from build123d import *

# Parameters (mm, degrees)
SKETCH_R        = 1.75
PAD_DEPTH       = 3.05
SKETCH001_W     = 60.21645
SKETCH001_H     = 13.401505
POCKET_DEPTH    = 2.9
POCKET001_DEPTH = 3.051
POCKET002_DEPTH = 36.525
FILLET_R        = 6


with BuildPart() as part:
    # Sketch → Pad (new body)
    with BuildSketch(Plane.XY):
        Polygon((-30, 0), (30, 0), (30, 12.7), (6.524, 12.7), (6.524, 19.05), (2.968, 19.05), (2.968, 12.7), (1.778, 12.7), (1.778, 19.05), (-1.778, 19.05), (-1.778, 12.7), (-2.968, 12.7), (-2.968, 19.05), (-6.524, 19.05), (-6.524, 12.7), (-30, 12.7), align=None)
        with Locations((-24, 6.35)):
            Circle(SKETCH_R, mode=Mode.SUBTRACT)
        with Locations((24, 6.35)):
            Circle(SKETCH_R, mode=Mode.SUBTRACT)
    extrude(amount=PAD_DEPTH)

    # Sketch001 (on Face20 of Pad) → Pocket (cut)
    with BuildSketch(Plane.XY.offset(3.05)):
        with Locations((-0.108225, 5.999248)):
            Rectangle(SKETCH001_W, SKETCH001_H)
    extrude(amount=-POCKET_DEPTH, mode=Mode.SUBTRACT)

    # Sketch002 (on Face25 of Pocket) → Pocket001 (cut, through all)
    with BuildSketch(Plane.XY.offset(3.05)):
        with BuildLine():
            ThreePointArc((-2.968, 17.272), (-4.746, 19.05), (-6.524, 17.272))
            Line((-6.524, 17.272), (-7.554864, 19.132154))
            Line((-7.554864, 19.132154), (-6.342233, 20.53426))
            Line((-6.342233, 20.53426), (5.632503, 20.53426))
            Line((5.632503, 20.53426), (7.211451, 19.637419))
            Line((6.524, 17.272), (7.211451, 19.637419))
            ThreePointArc((6.524, 17.272), (4.746, 19.05), (2.968, 17.272))
            Line((2.968, 17.272), (1.778, 17.272))
            ThreePointArc((1.778, 17.272), (0, 19.05), (-1.778, 17.272))
            Line((-1.778, 17.272), (-2.968, 17.272))
        make_face()
    extrude(amount=-POCKET001_DEPTH, mode=Mode.SUBTRACT)

    # Sketch003 (on Face7 of Pocket001) → Pocket002 (cut, through all)
    with BuildSketch(Plane(origin=(-6.524, 0, 0), x_dir=(0, -1, 0), z_dir=(-1, 0, 0))):
        with BuildLine():
            Line((-12.816161, 0), (-12.862388, -0.39199))
            Line((-12.862388, -0.39199), (-19.923561, -0.39199))
            Line((-19.923561, -0.39199), (-19.923561, 4.294415))
            Line((-19.923561, 4.294415), (-11.624612, 3.801784))
            Line((-11.624612, 3.801784), (-12.7, 0.15))
            ThreePointArc((-13.25543, 0.582616), (-13.017245, 0.315556), (-12.7, 0.15))
            ThreePointArc((-13.25543, 0.582616), (-16.088623, 2.498132), (-18.990517, 0.68838))
            Line((-18.799929, 0.68838), (-18.990517, 0.68838))
            ThreePointArc((-13.404078, 0.493377), (-16.039328, 2.325158), (-18.799929, 0.68838))
            ThreePointArc((-13.404078, 0.493377), (-13.14319, 0.207281), (-12.816161, 0))
        make_face()
    extrude(amount=-POCKET002_DEPTH, mode=Mode.SUBTRACT)

    # Fillet
    fillet_edges = [part.edges().sort_by_distance(p)[0] for p in [
        (30, 0, 0.075),
        (30, 12.7, 0.075),
        (-30, 12.7, 0.075),
        (-30, 0, 0.075),
    ]]
    fillet(fillet_edges, radius=FILLET_R)


solid = part.part
Geometry check sheet. Reference: the model listing, model coordinates, mm. Give positions to 0.01 mm unless a question says otherwise; leave off trailing zeros. Order: outer loops, then holes, each group sorted by start corner. A loop starts at its lowest first (then second) coordinate and runs counter-clockwise, first axis right, second up.
1) Gauge pin test, flat ends, axial feed: pin 1 (10 mm diameter, centred on x = 6.5, y = 6, fed in from +Z); pin 2 (1 mm diameter, centred on y = 5, z = 0.5, fed in from -X). Record the tip position at first contact, or that the pin passes through.
Results are:
pin 1: stops at z = 0.15
pin 2: stops at x = -29.97
2) Cross-section at A-A (z = 1.1). Record the boundary of the cut face in (x, y), then the cut area to 3 significant figures.
Results are:
outline: (-6.52, 13.53) - (-2.97, 13.53) - (-2.97, 13.74) - (-6.52, 13.74) - close; (-5.98, 18.55) - (-3.51, 18.55) arc R1.78 ccw to (-3.77, 18.76) - (-5.72, 18.76) arc R1.78 ccw to start; (-1.78, 13.53) - (1.78, 13.53) - (1.78, 13.74) - (-1.78, 13.74) - close; (-1.24, 18.55) - (1.24, 18.55) arc R1.78 ccw to (0.97, 18.76) - (-0.97, 18.76) arc R1.78 ccw to start; (2.97, 13.53) - (6.52, 13.53) - (6.52, 13.74) - (2.97, 13.74) - close; (3.51, 18.55) - (5.98, 18.55) arc R1.78 ccw to (5.72, 18.76) - (3.77, 18.76) arc R1.78 ccw to start
area: 3.62 mm2
3) Cross-section at D-D (y = 10). Record the boundary of the cut face in (x, z), then the cut area to 3 significant figures.
Results are:
outline: (-29.01, 0) - (29.01, 0) - (29.01, 0.15) - (-29.01, 0.15) - close
area: 8.70 mm2
4) Cross-section at C-C (x = 7.5). Record the boundary of the cut face in (y, z), then the cut area to 4 significant figures.
Results are:
outline: (0, 0) - (12.7, 0) - (12.7, 0.15) - (0, 0.15) - close
area: 1.905 mm2
5) Material ranges on probe 1 along X at (y, z) = (6.35, 0.1); probe 2 along Y at (x, z) = (24, 0.1); probe 3 along Y at (x, z) = (-1.5, 2.05), recorded low to high.
Results are:
probe 1: x = -30 to -25.75, -22.25 to 22.25, 25.75 to 30
probe 2: y = 0 to 4.6, 8.1 to 12.7
probe 3: y = 14.53 to 14.89, 17.4 to 17.76
6) Cross-section at B-B (y = 14.25). Record the boundary of the cut face in (x, z), then the cut area to 3 significant figures.
Results are:
outline: (-6.52, 1.64) - (-2.97, 1.64) - (-2.97, 1.86) - (-6.52, 1.86) - close; (-1.78, 1.64) - (1.78, 1.64) - (1.78, 1.86) - (-1.78, 1.86) - close; (2.97, 1.64) - (6.52, 1.64) - (6.52, 1.86) - (2.97, 1.86) - close
area: 2.34 mm2
